Autodesk Inventor part; units mm, degrees
ref_plane "YZ Plane" through (0, 0, 0) normal (1, 0, 0) x (0, 1, 0)
ref_plane "XZ Plane" through (0, 0, 0) normal (0, 1, 0) x (-1, 0, 0)
ref_plane "XY Plane" through (0, 0, 0) normal (0, 0, 1) x (1, 0, 0)
sketch "Esquisse1" plane through (0, 0, 0) normal (1, 0, 0) x (0, 1, 0)
  line L0 (-2.5, 65) -> (2.5, 65)
  line L1 (2.5, 65) -> (2.5, -65)
  line L2 (2.5, -65) -> (-2.5, -65)
  line L3 (-2.5, -65) -> (-2.5, 65)
  line L4 (2.5, 65) -> (-2.5, -65)
  line L5 (2.5, -65) -> (-2.5, 65)
  point P0 (0, 0)
  point P1 (0, 0)
  point P2 (0, 0)
  dimension "d0" = 130
  dimension "d1" = 5
extrude "Extrusion1" add sketch "Esquisse1" along normal blind 5
sketch "Esquisse2" plane through (5, 0, 0) normal (1, 0, 0) x (0, 0, -1)
  line L0 (65, 2.5) -> (-65, 2.5)
  line L1 (-65, -2.5) -> (65, -2.5)
  line L2 (-30, 2.5) -> (-20, 2.5)
  line L3 (-20, 2.5) -> (-20, -2.5)
  line L4 (-20, -2.5) -> (-30, -2.5)
  line L5 (-30, -2.5) -> (-30, 2.5)
  line L6 (0, 13) -> (0, -16)
  line L7 (30, 2.5) -> (20, 2.5)
  line L8 (20, 2.5) -> (20, -2.5)
  line L9 (20, -2.5) -> (30, -2.5)
  line L10 (30, -2.5) -> (30, 2.5)
  point P0 (0, 0)
  point P1 (-20, 2.5)
  point P2 (30, -2.5)
  point P3 (30, 2.5)
  point P4 (20, 2.5)
  point P5 (20, -2.5)
  dimension "d4" = 10
  dimension "d5" = 20
extrude "Extrusion2" add sketch "Esquisse2" along normal blind 10 contours L10 L1 L8 L0 | L3 L1 L5 L0
sketch "Esquisse3" plane through (0, 2.5, 65) normal (0, 1, 0) x (1, 0, 0)
  line L0 (15, 45) -> (15, 35)
  line L1 (5, 45) -> (15, 45)
  line L2 (15, 35) -> (12, 35)
  line L3 (12, 35) -> (12, 45)
  line L4 (12, 45) -> (15, 45)
  line L5 (15, 45) -> (15, 35)
  line L6 (-9, 65) -> (24, 65)
  line L7 (15, 85) -> (15, 95)
  line L8 (15, 95) -> (12, 95)
  line L9 (12, 95) -> (12, 85)
  line L10 (12, 85) -> (15, 85)
  line L11 (15, 85) -> (15, 95)
  point P0 (0, 65)
extrude "Extrusion3" add sketch "Esquisse3" along normal blind 10
sketch "Esquisse4" plane through (15, 0, 0) normal (1, 0, 0) x (0, 0, -1)
  circle A0 centre (-25, 8.5) radius 1.75
  line L0 (0, 20) -> (0, -21)
  circle A1 centre (25, 8.5) radius 1.75
  line L1 (-30, 12.5) -> (-20, 12.5)
  line L2 (-20, -2.5) -> (-20, 12.5)
  point P0 (0, 0)
  dimension "d10" = 3.5
  dimension "d11" = 4
  dimension "d19" = 5
extrude "Extrusion4" cut sketch "Esquisse4" against normal blind 10
fillet "Congé1" radius 5 4 edges at (5, 0, 30) (5, 0, -20) (5, 0, 20) (5, 0, -30)
fillet "Congé2" radius 3 2 edges at (15, -2.5, 25) (15, -2.5, -25)
fillet "Congé3" radius 3 2 edges at (5, 0, -65) (5, 0, 65)
sketch "Esquisse5" plane through (0, 0, 0) normal (-1, 0, 0) x (0, 0, 1)
  line L0 (-65, 2.5) -> (65, 2.5)
  line L1 (65, -2.5) -> (-65, -2.5)
  line L2 (-65, 2.5) -> (-62, 2.5)
  line L3 (-62, 2.5) -> (-62, -2.5)
  line L4 (-62, -2.5) -> (-65, -2.5)
  line L5 (-65, -2.5) -> (-65, 2.5)
  line L6 (0, 19) -> (0, -21)
  line L7 (65, 2.5) -> (62, 2.5)
  line L8 (62, 2.5) -> (62, -2.5)
  line L9 (62, -2.5) -> (65, -2.5)
  line L10 (65, -2.5) -> (65, 2.5)
  point P0 (0, 0)
  point P1 (65, -2.5)
extrude "Extrusion5" add sketch "Esquisse5" along normal blind 10 contours L0 L3 L1 L5 | L0 L10 L1 L8
properties part number "pare-chocs"
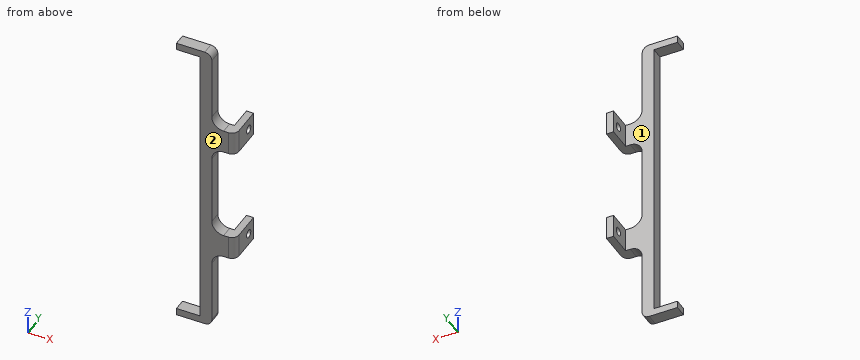
Model file for the job. Use its own axes, mm. Face numbers are marked on the shaded views. A direction names the side the tool comes from. Give positions to 0.01 mm unless a question says otherwise; leave off trailing zeros. Write each loop counter-clockwise with the first axis right and the second up, starting at its lowest first coordinate (ties: lowest second). Pieces come first, ordered by that corner, then holes. Notation, with made-up numbers: (80, 45.5) -> (101, 45.5) arc R12 cw to (101, 52.5) -> close; hole circle Ø4 at (-5, 59). An arc over 180 degrees is marked (long way). Use CSV: the item, a comma, the result in double quotes. Start each with the question number.
1) Cut at D-D on z = -3. List the corners of the cut face in (x, y).
2) Drill centre lines: L1, parallel to X at y = -1.5, z = 59; L2, parallel to Y at x = 13.8, z = 25; L3, parallel to Y at x = 14.1, z = 25. Where is each one in solid material? Low to high.
3) Cut at C-C on y = 8.5. List the corners of the cut face in (x, z), plus the area to 3 significant figures.
4) Pin check, flat tips, straight feed: P1, Ø8, axis at x = 5.5, y = 8.5, coming from the +Z side; P2, Ø2, axis at x = 4.5, z = 45, coming from the +Y side; P3, Ø5, axis at y = 1.5, z = 4.5, coming from the +X side; P4, Ø5.5, axis at x = 11.5, y = 4, coming from the -Z side. Stop position of each tip, or through.
5) Cut at B-B on x = -5. List the corners of the cut face in (y, z).
6) Cut at A-A on z = 25. List the corners of the cut face in (x, y).
7) Tool access for the marked faces 1 and 2: list every direction of +Z, -Z, +X, -X, +Y, -Y with a clear straight run to the whole face (end or side of a thin tool).
Final values:
1,outline,"(0, -2.5) -> (5, -2.5) -> (5, 2.5) -> (0, 2.5) -> close"
2,L1,"x = 0 to 5"
2,L2,"y = -1.9 to 6.75, 10.25 to 12.5"
2,L3,"y = -1.64 to 6.75, 10.25 to 12.5"
3,outline,"(12, -30) -> (15, -30) -> (15, -26.75) -> (12, -26.75) -> close; (12, -23.25) -> (15, -23.25) -> (15, -20) -> (12, -20) -> close; (12, 20) -> (15, 20) -> (15, 23.25) -> (12, 23.25) -> close; (12, 26.75) -> (15, 26.75) -> (15, 30) -> (12, 30) -> close"
3,area,"39.0 mm2"
4,P1,"passes through"
4,P2,"stops at y = 2.5"
4,P3,"stops at x = 5"
4,P4,"stops at z = -30.07"
5,outline,"(-2.5, -65) -> (2.5, -65) -> (2.5, -62) -> (-2.5, -62) -> close; (-2.5, 62) -> (2.5, 62) -> (2.5, 65) -> (-2.5, 65) -> close"
6,outline,"(0, -2.5) -> (12, -2.5) arc R3 ccw to (15, 0.5) -> (15, 6.75) -> (12, 6.75) -> (12, 2.5) -> (0, 2.5) -> close; (12, 10.25) -> (15, 10.25) -> (15, 12.5) -> (12, 12.5) -> close"
7,face 1,"+Z, -Z, -X, +Y"
7,face 2,"+Z, -Z, +X, -X, -Y"
